Check sheet for the drawn part. Datum: minimum x, y, z corner. Units: mm. A direction names the side the tool comes from. Round coordinates to 2 decimals unless told otherwise and drop trailing zeros. Write each loop counter-clockwise with the first axis right and the second up, starting at its lowest first coordinate (ties: lowest second). Pieces come first, ordered by that corner, then holes. Notation, with made-up numbers: (28, -20) -> (54, -20) arc R6 ccw to (54, -15) -> close; hole circle Ø1 at (12, -24). An arc over 180 degrees is marked (long way). Use a Markdown table: item, result.
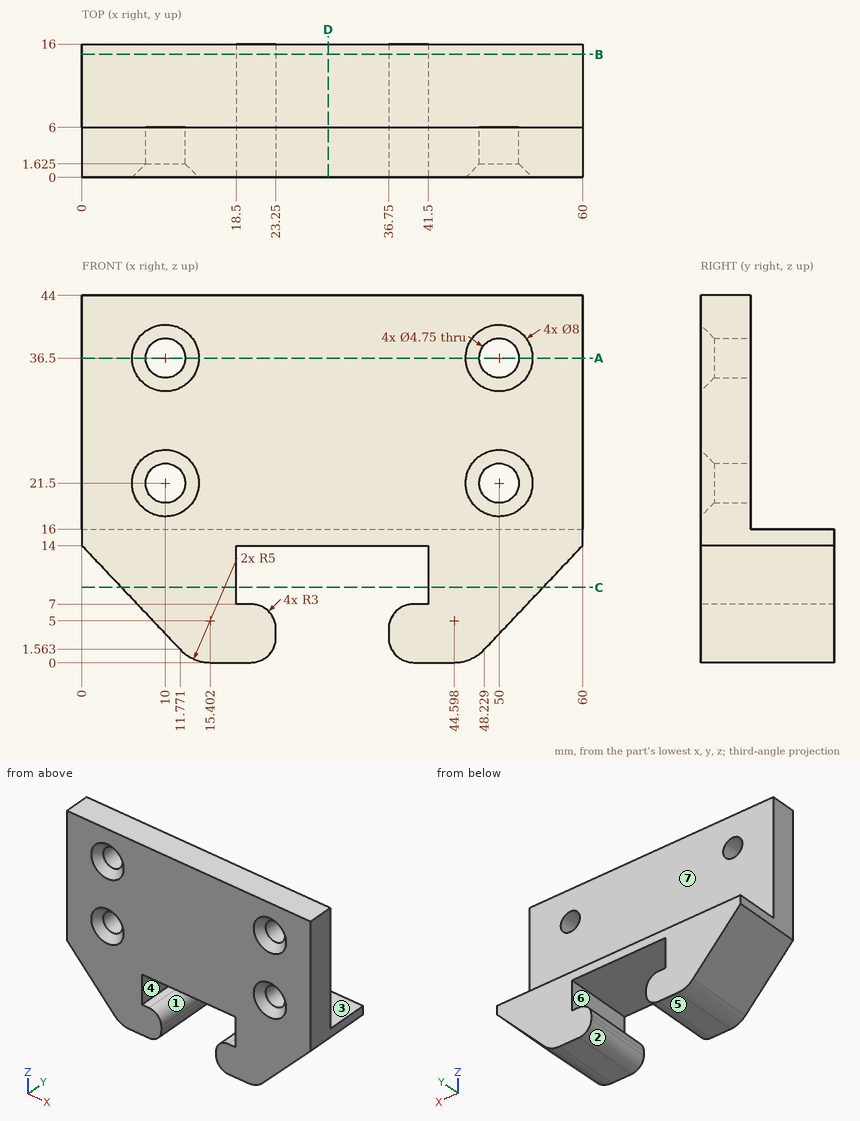
(1) Section check B-B on y = 14.75. Record the cut outline in (x, z).
A:
| item | result |
|---|---|
| outline | (0, 14) -> (11.77, 1.56) arc R5 ccw to (15.4, 0) -> (20.25, 0) arc R3 ccw to (23.25, 3) -> (23.25, 4) arc R3 ccw to (20.25, 7) -> (18.5, 7) -> (18.5, 14) -> (41.5, 14) -> (41.5, 7) -> (39.75, 7) arc R3 ccw to (36.75, 4) -> (36.75, 3) arc R3 ccw to (39.75, 0) -> (44.6, 0) arc R5 ccw to (48.23, 1.56) -> (60, 14) -> (60, 16) -> (0, 16) -> close |
(2) Section check C-C on z = 9. Record the cut outline in (x, y).
A:
| item | result |
|---|---|
| outline | (4.73, 0) -> (18.5, 0) -> (18.5, 16) -> (4.73, 16) -> close; (41.5, 0) -> (55.27, 0) -> (55.27, 16) -> (41.5, 16) -> close |
(3) Release check for a two-part mould opening along Z. For the marked faces 4, 5, 6 and 7 record: +Z half, -Z half, draft (parallel to the pull), parting line (faces both ways), or undercut.
A:
| item | result |
|---|---|
| face 4 | undercut |
| face 5 | -Z half |
| face 6 | undercut |
| face 7 | draft |
(4) Thickness scan on line 1 (X direction, y = 3.45, z = 21.5) (1 decimal); line 2 (Z direction, x = 39.5, y = 8); line 3 (Z direction, x = 50, y = 4.65) (1 decimal). Record the ranges inside material, lowest first.
A:
| item | result |
|---|---|
| line 1 | x = 0 to 7.6, 12.4 to 47.6, 52.4 to 60 |
| line 2 | z = 0.01 to 6.99, 14 to 16 |
| line 3 | z = 3.4 to 19.1, 23.9 to 34.1, 38.9 to 44 |
(5) Section check A-A on z = 36.5. Record the cut outline in (x, y) (1 decimal), plus the area to 3 significant figures.
A:
| item | result |
|---|---|
| outline | (0, 0) -> (6, 0) -> (7.6, 1.6) -> (7.6, 6) -> (0, 6) -> close; (12.4, 1.6) -> (14, 0) -> (46, 0) -> (47.6, 1.6) -> (47.6, 6) -> (12.4, 6) -> close; (52.4, 1.6) -> (54, 0) -> (60, 0) -> (60, 6) -> (52.4, 6) -> close |
| area | 298 mm2 |
(6) Access from +Z, -Z, +X, -X, +Y, -Y to the whole of each face (thin tool, end or side, straight path). Record for the marked faces 1, 2 and 3.
A:
| item | result |
|---|---|
| face 1 | +Y, -Y |
| face 2 | -Z, +Y, -Y |
| face 3 | +Z, +X, -X, +Y |
(7) Gauge pin test, flat ends, axial feed: pin 1 Ø5 at (x, y) = (21, 10.5) entering from +Z; pin 2 Ø0.8 at (y, z) = (5.5, 3.5) entering from +X; pin 3 Ø5 at (x, z) = (27.5, 22.5) entering from +Y. Record the tip position at first contact, or that the pin passes through.
A:
| item | result |
|---|---|
| pin 1 | stops at z = 16 |
| pin 2 | stops at x = 50.44 |
| pin 3 | stops at y = 6 |
(8) Section check D-D on x = 29.5. Record the cut outline in (y, z).
A:
| item | result |
|---|---|
| outline | (0, 14) -> (16, 14) -> (16, 16) -> (6, 16) -> (6, 44) -> (0, 44) -> close |
